from build123d import *

# Parameters (mm, degrees)
EXTRUDE1_DEPTH         = 15
SKETCH2_R              = 30
F_60_UDBORINGER_DEPTH  = 16
SKETCH3_R              = 7
M16_GEVINDHULLER_DEPTH = 16


with BuildPart() as part:
    # Sketch1 → Extrude1 (new body)
    with BuildSketch(Plane.XY):
        with BuildLine():
            Line((-250, 70), (-240, 70))
            ThreePointArc((-240, 70), (-229.653341221, 69.231110435), (-219.533980669, 66.941332917))
            Line((-219.533980669, 66.941332917), (-149.757667724, 45.608573211))
            ThreePointArc((-149.757667724, 45.608573211), (-106.388979647, 35.795240991), (-62.046156308, 32.5))
            Line((-62.046156308, 32.5), (62.046156308, 32.5))
            ThreePointArc((62.046156308, 32.5), (106.388979647, 35.795240991), (149.757667724, 45.608573211))
            Line((149.757667724, 45.608573211), (219.533980669, 66.941332917))
            ThreePointArc((219.533980669, 66.941332917), (229.653341221, 69.231110435), (240, 70))
            Line((240, 70), (250, 70))
            ThreePointArc((250, 70), (320, 0), (250, -70))
            Line((250, -70), (240, -70))
            ThreePointArc((240, -70), (229.653341221, -69.231110435), (219.533980669, -66.941332917))
            Line((219.533980669, -66.941332917), (149.757667724, -45.608573211))
            ThreePointArc((149.757667724, -45.608573211), (106.388979647, -35.795240991), (62.046156308, -32.5))
            Line((62.046156308, -32.5), (-62.046156308, -32.5))
            ThreePointArc((-62.046156308, -32.5), (-106.388979647, -35.795240991), (-149.757667724, -45.608573211))
            Line((-149.757667724, -45.608573211), (-219.533980669, -66.941332917))
            ThreePointArc((-219.533980669, -66.941332917), (-229.653341221, -69.231110435), (-240, -70))
            Line((-240, -70), (-250, -70))
            ThreePointArc((-250, -70), (-320, 0), (-250, 70))
        make_face()
    extrude(amount=EXTRUDE1_DEPTH)

    # Sketch2 → ø60 udboringer (cut, through all)
    with BuildSketch(Plane.XY.offset(15)):
        with Locations((245, 0)):
            Circle(SKETCH2_R)
        with Locations((-245, 0)):
            Circle(SKETCH2_R)
    extrude(amount=-F_60_UDBORINGER_DEPTH, mode=Mode.SUBTRACT)

    # Sketch3 → M16 gevindhuller (cut, through all)
    with BuildSketch(Plane.XY.offset(15)):
        with Locations((160, 0)):
            Circle(SKETCH3_R)
        with Locations((-160, 0)):
            Circle(SKETCH3_R)
    extrude(amount=-M16_GEVINDHULLER_DEPTH, mode=Mode.SUBTRACT)


solid = part.part
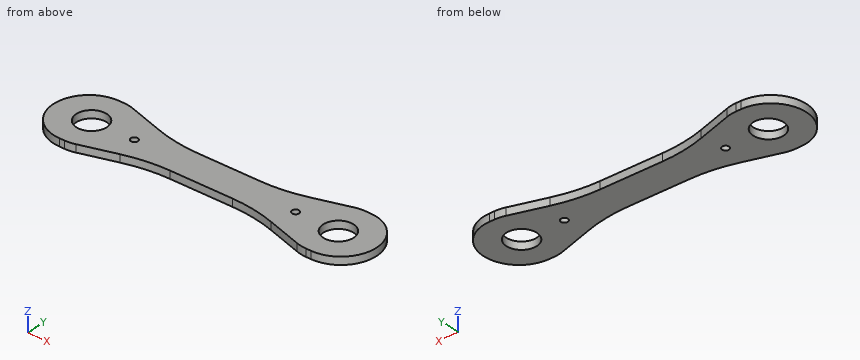
Model file for the job. Use its own axes, mm. Round coordinates to 2 decimals unless told otherwise and drop trailing zeros. Loops run counter-clockwise (first coordinate to the right, second up) from the corner with the lowest first, then second, coordinate; pieces in that order, holes last. Notation, with made-up numbers: (61, -15) - (92, -15) arc R26 ccw to (92, 17) - close; hole circle Ø11 at (4, -35). An arc over 180 degrees is marked (long way). Write each question's results on one line, items separated by ' | '.
(1) Saw through at C-C, the plane z = 11.75. List the corners of the cut face in (x, y), then the cut area to 3 significant figures.
Answer below:
outline: (-250, -70) - (-240, -70) arc R70 ccw to (-219.53, -66.94) - (-149.76, -45.61) arc R300 cw to (-62.05, -32.5) - (62.05, -32.5) arc R300 cw to (149.76, -45.61) - (219.53, -66.94) arc R70 ccw to (240, -70) - (250, -70) arc R70 ccw to (250, 70) - (240, 70) arc R70 ccw to (219.53, 66.94) - (149.76, 45.61) arc R300 cw to (62.05, 32.5) - (-62.05, 32.5) arc R300 cw to (-149.76, 45.61) - (-219.53, 66.94) arc R70 ccw to (-240, 70) - (-250, 70) arc R70 ccw to start; hole circle Ø60 at (-245, 0); hole circle Ø14 at (-160, 0); hole circle Ø14 at (160, 0); hole circle Ø60 at (245, 0) | area: 54,600 mm^2
(2) Pin check, flat tips, straight feed: pin 1 (22.5 mm diameter, centred on x = -160, y = 0, fed in from +Z); pin 2 (1 mm diameter, centred on x = -139, z = 8, fed in from -Y); pin 3 (1 mm diameter, centred on y = -30, z = 9, fed in from +X); pin 4 (2 mm diameter, centred on y = -13, z = 12.5, fed in from +X). Stop position of each tip, or through.
Answer below:
pin 1: stops at z = 15 | pin 2: stops at y = -42.67 | pin 3: stops at x = 313.48 | pin 4: stops at x = 318.96
(3) Saw through at B-B, the plane x = -160. List the corners of the cut face in (y, z), then the cut area to 3 significant figures.
Answer below:
outline: (-48.74, 0) - (-7, 0) - (-7, 15) - (-48.74, 15) - close; (7, 0) - (48.74, 0) - (48.74, 15) - (7, 15) - close | area: 1,250 mm^2
(4) Saw through at A-A, the plane y = 0. List the corners of the cut face in (x, z), then the cut area to 3 significant figures.
Answer below:
outline: (-320, 0) - (-275, 0) - (-275, 15) - (-320, 15) - close; (-215, 0) - (-167, 0) - (-167, 15) - (-215, 15) - close; (-153, 0) - (153, 0) - (153, 15) - (-153, 15) - close; (167, 0) - (215, 0) - (215, 15) - (167, 15) - close; (275, 0) - (320, 0) - (320, 15) - (275, 15) - close | area: 7,380 mm^2
(5) Wall check: L1, parallel to Y at x = 245, z = 8.5; L2, parallel to X at y = -21.5, z = 7; L3, parallel to Y at x = -19, z = 3.5. Give the ranges that are in metal, low to high.
Answer below:
L1: y = -70 to -30, 30 to 70 | L2: x = -316.62 to -265.92, -224.08 to 224.08, 265.92 to 316.62 | L3: y = -32.5 to 32.5
(6) Saw through at D-D, the plane y = 24. List the corners of the cut face in (x, z).
Answer below:
outline: (-315.76, 0) - (-263, 0) - (-263, 15) - (-315.76, 15) - close; (-227, 0) - (227, 0) - (227, 15) - (-227, 15) - close; (263, 0) - (315.76, 0) - (315.76, 15) - (263, 15) - close
